```python
from build123d import *

# Parameters (mm, degrees)
F0_W     = 88.9
F0_H     = 88.9
F1_DEPTH = 3.175
F3_D     = 38.15


with BuildPart() as f1:
    # F0 (on Right) → F1 (new body, symmetric)
    with BuildSketch(Plane.YZ):
        with Locations((1.86388e-05, 0)):
            Rectangle(F0_W, F0_H)
    extrude(amount=F1_DEPTH, both=True)

    # F3 (through all)
    with Locations(Plane(origin=(-3.175, 0, 0), x_dir=(0, -1, 0), z_dir=(-1, 0, 0))):
        with Locations((-1.86388e-05, 0)):
            Hole(F3_D / 2)


solid = f1.part
```
The listing builds one solid part. Answer for the finished solid, in the listing's coordinates (mm). Coordinates: 2 decimals unless noted, no trailing zeros. Loops run counter-clockwise (first coordinate to the right, second up) from the corner with the lowest first, then second, coordinate; pieces in that order, holes last. Notation, with made-up numbers: (-3.5, -12.5) - (55.5, -12.5) arc R19 cw to (55.5, 11.5) - close; hole circle Ø6 at (39, -23.5). An arc over 180 degrees is marked (long way). Use a Markdown table: item, result. Add a question column.
1) Find the intervals of material crossed by line 1 (Z direction, x = -0.5, y = 15); line 2 (Z direction, x = 2, y = 2); line 3 (Y direction, x = 1.75, z = 6.5), in increasing order.
2) The part is cut by section B-B, the plane z = 0. Give the vertices of the cut face in (x, y) (3 decimals).
3) The mould has two halves that part along Z. Classify faces 1 (the flat face through (0, -1, -44.45)), 2 (the cylindrical face through (0.044, 10.255, 16.084)), 3 (the flat face through (0, -1, 44.45)), 4 (the flat face through (0, 44.45, -1)): released by +Z, released by -Z, zero draft, split by the parting line, or undercut.
4) The part is cut by section C-C, the plane x = -1.25. Give the vertices of the cut face in (y, z) (3 decimals), and give its area (3 significant figures).
5) The part is cut by section A-A, the plane y = 4.5. Give the vertices of the cut face in (x, z) (3 decimals), and give its area (3 significant figures).
Here are the results:
| question | item | result |
|---|---|---|
| 1 | line 1 | z = -44.45 to -11.78, 11.78 to 44.45 |
| 1 | line 2 | z = -44.45 to -18.97, 18.97 to 44.45 |
| 1 | line 3 | y = -44.45 to -17.93, 17.93 to 44.45 |
| 2 | outline | (-3.175, -44.45) - (3.175, -44.45) - (3.175, -19.075) - (-3.175, -19.075) - close; (-3.175, 19.075) - (3.175, 19.075) - (3.175, 44.45) - (-3.175, 44.45) - close |
| 3 | face 1 | released by -Z |
| 3 | face 2 | undercut |
| 3 | face 3 | released by +Z |
| 3 | face 4 | zero draft |
| 4 | outline | (-44.45, -44.45) - (44.45, -44.45) - (44.45, 44.45) - (-44.45, 44.45) - close; hole circle Ø38.15 at (0, 0) |
| 4 | area | 6,760 mm^2 |
| 5 | outline | (-3.175, -44.45) - (3.175, -44.45) - (3.175, -18.537) - (-3.175, -18.537) - close; (-3.175, 18.537) - (3.175, 18.537) - (3.175, 44.45) - (-3.175, 44.45) - close |
| 5 | area | 329 mm^2 |
